from build123d import *

# Parameters (mm, degrees)
EXTRUDE_1_DEPTH      = 10
EXTRUDE_2_DEPTH      = 11
EXTRUDE_2_DEPTH_BACK = 16.5
CUT_EXTRUDE_1_DEPTH  = 28.5
HOLE_WIZARD_M3_1_D   = 2.5


with BuildPart() as part:
    # 스케치1 → 보스-돌출1 (new body)
    with BuildSketch(Plane.XY):
        with BuildLine():
            Line((6.577848346, 2.394141003), (86.577848346, -11.712017453))
            Line((86.577848346, -11.712017453), (85.759003896, -16.355915091))
            Line((85.759003896, -16.355915091), (6.577848346, -2.394141003))
            ThreePointArc((6.577848346, -2.394141003), (-7, 0), (6.577848346, 2.394141003))
        make_face()
    extrude(amount=EXTRUDE_1_DEPTH)

    # 스케치2 → 보스-돌출2 (add, two sides)
    with BuildSketch(Plane.XY.offset(10)) as extrude_2_sk:
        Polygon((86.577848346, -11.712017453), (27.489383165, -1.293126793), (26.670538716, -5.937024431), (85.759003896, -16.355915091), align=None)
    extrude(amount=EXTRUDE_2_DEPTH)
    extrude(extrude_2_sk.sketch, amount=-EXTRUDE_2_DEPTH_BACK)

    # 스케치4 → 컷-돌출1 (cut, through all)
    with BuildSketch(Plane.XY.offset(21)):
        Polygon((86.577848346, -11.712017453), (85.759003896, -16.355915091), (37.556934536, -3.06830773), align=None)
    extrude(amount=-CUT_EXTRUDE_1_DEPTH, mode=Mode.SUBTRACT)

    # M3 나사 구멍1 (through all)
    with Locations(Plane.XY.offset(10)):
        with Locations((-4, 0), (0, 4), (4, 0), (0, -4)):
            Hole(HOLE_WIZARD_M3_1_D / 2)


solid = part.part
Verification items for the finished model (mm, model axes). A direction names the side the tool comes from. Coordinates: 2 decimals unless noted, no trailing zeros. Write each loop counter-clockwise with the first axis right and the second up, starting at its lowest first coordinate (ties: lowest second). Pieces come first, ordered by that corner, then holes. Notation, with made-up numbers: (-15, 57.25) -> (33, 57.25) arc R24 ccw to (33, 86.25) -> close; hole circle Ø7 at (0.25, -8.75). An arc over 180 degrees is marked (long way). One line per item, written item: value. Start each with the question number.
Q1. Cross-section at A-A on z = 5.5. Enter the section's corners in (x, y), and give its area (3 significant figures).
Q2. Access from +Z, -Z, +X, -X, +Y, -Y to the whole of each face (thin tool, end or side, straight path). Record for faces 1 (the flat face through (27.086, -3.583, 15.423)), 2 (the flat face through (27.086, -3.583, -3.204)), 3 (the cylindrical face through (-5.19, 0.38, 4.93)).
Q3. Thickness scan on L1, parallel to Y at x = 0, z = 4.25; L2, parallel to Y at x = 4, z = 7.25; L3, parallel to Z at x = 12.5, y = -1.5. Record the ranges inside material, lowest first. Write a range as from..to.
Q4. Cross-section at C-C on x = 0. Enter the section's corners in (y, z), and give its area (3 significant figures).
Q5. Cross-section at D-D on y = 0. Enter the section's corners in (x, z).
Q6. Mould release check, pull along Y, two halves, no side actions. Record for faces 4 (the cylindrical face through (5.25, 0.05, 4.93)), 5 (the cylindrical face through (-7, 0, 5)), 6 (the flat face through (7, 0, 0)): pulls with the +Y half, pulls with the -Y half, needs draft (parallel to the pull), parting line crosses it, or undercut.
Q7. Cross-section at B-B on y = 4. Enter the section's corners in (x, z).
Q8. Go/stop test with flat-tipped pins: P1, Ø8, axis at x = 54.5, z = 9.5, coming from the -Y side; P2, Ø1.5, axis at x = 36, z = 15.5, coming from the -Y side; P3, Ø11, axis at x = 12.5, y = 1.5, coming from the -Z side. Record where each tip stops, or that it passes through.
Checked values:
1. outline: (6.58, -2.39) -> (85.76, -16.36) -> (37.56, -3.07) -> (6.58, 2.39) arc R7 ccw (long way) to start; hole circle Ø2.5 at (-4, 0); hole circle Ø2.5 at (0, -4); hole circle Ø2.5 at (0, 4); hole circle Ø2.5 at (4, 0)
1. area: 397 mm²
2. face 1: +Z, -X, +Y
2. face 2: -Z, -X, +Y
2. face 3: +Z, -Z
3. L1: y = -7..-5.25, -2.75..2.75, 5.25..7
3. L2: y = -5.74..-1.25, 1.25..5.74
3. L3: z = 0..10
4. outline: (-7, 0) -> (-5.25, 0) -> (-5.25, 10) -> (-7, 10) -> close; (-2.75, 0) -> (2.75, 0) -> (2.75, 10) -> (-2.75, 10) -> close; (5.25, 0) -> (7, 0) -> (7, 10) -> (5.25, 10) -> close
4. area: 90.0 mm²
5. outline: (-7, 0) -> (-5.25, 0) -> (-5.25, 10) -> (-7, 10) -> close; (-2.75, 0) -> (2.75, 0) -> (2.75, 10) -> (-2.75, 10) -> close; (5.25, 0) -> (20.16, 0) -> (20.16, 10) -> (5.25, 10) -> close
6. face 4: undercut
6. face 5: parting line crosses it
6. face 6: needs draft
7. outline: (-5.74, 0) -> (-1.25, 0) -> (-1.25, 10) -> (-5.74, 10) -> close; (1.25, 0) -> (5.74, 0) -> (5.74, 10) -> (1.25, 10) -> close
8. P1: stops at y = -11.55
8. P2: stops at y = -7.71
8. P3: stops at z = 0
